Read the model definition and answer for the solid it produces. Units are mm, in the model's axes. Coordinates: 2 decimals unless noted, no trailing zeros. Write each loop counter-clockwise with the first axis right and the second up, starting at its lowest first coordinate (ties: lowest second). Pieces come first, ordered by that corner, then holes. Notation, with made-up numbers: (20.25, -23.5) -> (42.25, -23.5) arc R22 ccw to (42.25, -17.5) -> close; hole circle Ø5 at (37.5, 88.5). An arc over 180 degrees is marked (long way). Write item = value, one per line. Start each with the question number.
1) Find the intervals of material crossed by line 1 along X through (y, z) = (66.5, 2.15) (3 decimals); line 2 along X through (y, z) = (6.35, 1.65) (3 decimals); line 3 along Y through (x, z) = (19, 1), in increasing order. Write a range as from..to.
2) Section A-A (y = 103.5) is taken. Determine the outline of the cut face in (x, z).
3) Flat-ended cylindrical pins translate along their axes: pin 1 Ø1 at (x, z) = (9, 0.5) entering from +Y; pin 2 Ø5 at (x, y) = (-3.175, 141.605) entering from -Z; pin 3 Ø1.5 at (x, z) = (20, 1.5) entering from +Y; pin 4 Ø0.9 at (y, z) = (60.5, 1.5) entering from -X. Find the tip coordinate at first contact, or state that the pin passes through.
4) Section B-B (x = 1.5) is taken. Determine the outline of the cut face in (y, z), plus the area to 3 significant figures.
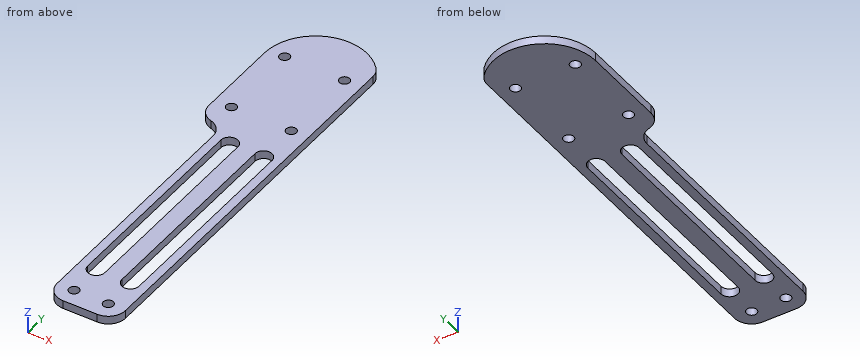
Autodesk Inventor part; units mm, degrees
ref_plane "YZ Plane" through (0, 0, 0) normal (1, 0, 0) x (0, 1, 0)
ref_plane "XZ Plane" through (0, 0, 0) normal (0, 1, 0) x (-1, 0, 0)
ref_plane "XY Plane" through (0, 0, 0) normal (0, 0, 1) x (1, 0, 0)
sketch "Sketch1" plane through (0, 0, 0) normal (0, 0, 1) x (1, 0, 0)
  line L0 (0, 0) -> (25.4, 0)
  line L1 (25.4, 0) -> (25.4, 101.6)
  line L2 (25.4, 101.6) -> (0, 101.6)
  line L3 (0, 101.6) -> (0, 0)
  line L4 (6.35, 95.25) -> (6.35, 19.05) construction
  line L5 (3.175, 95.25) -> (3.175, 19.05)
  line L6 (9.525, 19.05) -> (9.525, 95.25)
  arc A0 (9.525, 95.25) -> (3.175, 95.25) centre (6.35, 95.25) ccw
  arc A1 (3.175, 19.05) -> (9.525, 19.05) centre (6.35, 19.05) ccw
  line L7 (19.05, 95.25) -> (19.05, 19.05) construction
  line L8 (15.875, 95.25) -> (15.875, 19.05)
  line L9 (22.225, 19.05) -> (22.225, 95.25)
  arc A2 (22.225, 95.25) -> (15.875, 95.25) centre (19.05, 95.25) ccw
  arc A3 (15.875, 19.05) -> (22.225, 19.05) centre (19.05, 19.05) ccw
  line L10 (6.35, 57.15) -> (19.05, 57.15) construction
  point P0 (12.7, 57.15)
  point P1 (12.7, 0)
  dimension "d2" = 6.35
  dimension "d3" = 76.2
  dimension "d4" = 19.05
  dimension "d5" = 6.35
  dimension "d7" = 12.7
  dimension "d8" = 3.175
extrude "Plate1" add sketch "Sketch1" along normal blind 3.048
sketch "Sketch2" plane through (0, 0, 3.048) normal (0, 0, 1) x (1, 0, 0)
  arc A0 (25.4, 150.2303) -> (-9.525, 139.7) centre (9.525, 139.7) ccw
  line L0 (25.4, 0) -> (25.4, 101.6)
  line L1 (25.4, 101.6) -> (0, 101.6)
  line L2 (0, 101.6) -> (-9.525, 101.6)
  line L3 (-9.525, 101.6) -> (-9.525, 139.7)
  line L4 (25.4, 101.6) -> (25.4, 150.2303)
  point P0 (0, 0)
  point P1 (28.575, 139.7)
  dimension "d10" = 38.1
  dimension "d11" = 3.175
  dimension "d12" = 38.1
  dimension "d13" = 34.925
sheet face with bend "Face2" sketch "Sketch2" thickness 3.048 toward (0, 0, -1) bend radius 3.048
bend "Bend1"
fillet "Corner Round1" radius 6.35 5 edges at (-9.525, 101.6, 1.524) (0, 101.6, 1.524) (25.4, 150.2303, 1.524) (0, 0, 1.524) (25.4, 0, 1.524)
sketch "Sketch3" plane through (0, 0, 3.048) normal (0, 0, 1) x (1, 0, 0)
  line L0 (6.35, 6.35) -> (19.05, 6.35) construction
  line L1 (19.05, 0) -> (6.35, 0)
  line L2 (25.4, 148.1003) -> (25.4, 6.35)
  line L3 (-9.525, 139.7) -> (-9.525, 107.95)
  line L4 (-3.175, 111.125) -> (19.05, 111.125) construction
  line L5 (-9.525, 123.825) -> (25.4, 123.825) construction
  point P0 (0, 0)
  point P1 (12.7, 6.35)
  point P2 (12.7, 0)
  point P3 (19.05, 141.605)
  point P4 (-3.175, 141.605)
  point P5 (7.9375, 123.825)
  point P6 (7.9375, 111.125)
  dimension "d20" = 6.35
  dimension "d21" = 6.35
  dimension "d22" = 6.35
  dimension "d23" = 3.175
  dimension "d25" = 30.48
hole "Hole1" at (6.35, 6.35, 3.048) at (19.05, 6.35, 3.048) at (-3.175, 111.125, 3.048) at (19.05, 111.125, 3.048) at (19.05, 141.605, 3.048) at (-3.175, 141.605, 3.048) direction (0, 0, -1) diameter 3.81 end through all
equation "\"d31\" = Thickness"
equation "\"d9\" = Thickness"
equation "\"d14\" = BendRadius"
equation "\"d15\" = BendReliefWidth"
equation "\"d17\" = MinimumRemnant"
equation "\"d16\" = BendReliefDepth"
equation "\"d18\" = TransitionRadius"
equation "\"BendRadius\" = Thickness"
equation "\"BendReliefWidth\" = Thickness"
equation "\"BendReliefDepth\" = 0.5 * Thickness"
equation "\"CornerReliefSize\" = 4 * Thickness"
equation "\"MinimumRemnant\" = 2 * Thickness"
equation "\"TransitionRadius\" = BendRadius"
equation "\"JacobiRadiusSize\" = BendRadius"
equation "\"GapSize\" = Thickness"
properties part number "Side Plate"
Answer key:
q1.line_1 = 0..3.175, 9.525..15.875, 22.225..25.4
q1.line_2 = 0..4.445, 8.255..17.145, 20.955..25.4
q1.line_3 = 0..4.45, 8.25..15.88, 98.42..109.22, 113.03..139.7, 143.51..156.23
q2.outline = (-7.7, 0) -> (25.4, 0) -> (25.4, 3.05) -> (-7.7, 3.05) -> close
q3.pin_1 = 158.75
q3.pin_2 = 0
q3.pin_3 = 156.08
q3.pin_4 = 0
q4.outline = (2.25, 0) -> (156.98, 0) -> (156.98, 3.05) -> (2.25, 3.05) -> close
q4.area = 472 mm^2
